Geometry check sheet. Reference: the model listing, model coordinates, mm. A direction names the side the tool comes from. Give positions to 0.01 mm unless a question says otherwise; leave off trailing zeros. Loops run counter-clockwise (first coordinate to the right, second up) from the corner with the lowest first, then second, coordinate; pieces in that order, holes last. Notation, with made-up numbers: (16.5, 56.25) -> (27.5, 56.25) arc R12 ccw to (27.5, 67.25) -> close; hole circle Ø8 at (-30, 0.25). An arc over 180 degrees is marked (long way). Answer in a Markdown table with one row per item. Add a question column.
```python
from build123d import *

# Parameters (mm, degrees)
SKETCH_W  = 30
SKETCH_H  = 26
PAD_DEPTH = 7


with BuildPart() as part:
    # Sketch → Pad (new body)
    with BuildSketch(Plane.XY):
        with Locations((15, 13)):
            Rectangle(SKETCH_W, SKETCH_H)
        with BuildLine():
            ThreePointArc((25.2, 18.8), (22, 22), (18.8, 18.8))
            Line((18.8, 18.8), (18.8, 7.2))
            ThreePointArc((18.8, 7.2), (22, 4), (25.2, 7.2))
            Line((25.2, 18.8), (25.2, 7.2))
        make_face(mode=Mode.SUBTRACT)
    pad = extrude(amount=PAD_DEPTH)

    # Mirrored: Pad across Sketch V_Axis
    add(pad.mirror(Plane(origin=(0, 0, 0), x_dir=(0, 0, 1), z_dir=(1, 0, 0))))


solid = part.part
```
1. Sectioned sample at A-A (x = 22). Enter the section's corners in (y, z).
2. Release check for a two-part mould opening along X. For faces 3 (the face through (0, 0, 3)), 4 (the face through (-18.8, 13, 3)), 5 (the face through (30, 13, 3)), 6 (the face through (-30, 13, 3)) record: released by +X, released by -X, zero draft, split by the parting line, or undercut.
3. Gauge pin test, flat end, axial feed: pin 1 Ø6 at (x, y) = (-19, 19) entering from +Z. Record the tip position at first contact, or that the pin passes through.
4. Sectioned sample at B-B (y = 13). Enter the section's corners in (x, z).
5. Sectioned sample at C-C (z = 3.5). Enter the section's corners in (x, y), plus the area to 3 significant figures.
6. Sectioned sample at D-D (x = -24.5). Enter the section's corners in (y, z), plus the area to 3 significant figures.
7. Material ranges on L1, parallel to X at y = 18.25, z = 3; L2, parallel to X at y = 6.5, z = 4.75; L3, parallel to Y at x = 21, z = 5.5, recorded low to high. Write a range as from..to.
8. Access from +Z, -Z, +X, -X, +Y, -Y to the whole of each face (thin tool, end or side, straight path). Record for faces 1 (the face through (0, 26, 3)), 2 (the face through (-25.2, 13, 3)).
Response:
| question | item | result |
|---|---|---|
| 1 | outline | (0, 0) -> (4, 0) -> (4, 7) -> (0, 7) -> close; (22, 0) -> (26, 0) -> (26, 7) -> (22, 7) -> close |
| 2 | face 3 | zero draft |
| 2 | face 4 | undercut |
| 2 | face 5 | released by +X |
| 2 | face 6 | released by -X |
| 3 | pin 1 | stops at z = 7 |
| 4 | outline | (-30, 0) -> (-25.2, 0) -> (-25.2, 7) -> (-30, 7) -> close; (-18.8, 0) -> (18.8, 0) -> (18.8, 7) -> (-18.8, 7) -> close; (25.2, 0) -> (30, 0) -> (30, 7) -> (25.2, 7) -> close |
| 5 | outline | (-30, 0) -> (30, 0) -> (30, 26) -> (-30, 26) -> close; hole (-25.2, 7.2) arc R3.2 ccw to (-18.8, 7.2) -> (-18.8, 18.8) arc R3.2 ccw to (-25.2, 18.8) -> close; hole (18.8, 7.2) arc R3.2 ccw to (25.2, 7.2) -> (25.2, 18.8) arc R3.2 ccw to (18.8, 18.8) -> close |
| 5 | area | 1,350 mm2 |
| 6 | outline | (0, 0) -> (5.2, 0) -> (5.2, 7) -> (0, 7) -> close; (20.8, 0) -> (26, 0) -> (26, 7) -> (20.8, 7) -> close |
| 6 | area | 72.8 mm2 |
| 7 | L1 | x = -30..-25.2, -18.8..18.8, 25.2..30 |
| 7 | L2 | x = -30..-25.12, -18.88..18.88, 25.12..30 |
| 7 | L3 | y = 0..4.16, 21.84..26 |
| 8 | face 1 | +Z, -Z, +X, -X, +Y |
| 8 | face 2 | +Z, -Z |
